from build123d import *

# Parameters (mm, degrees)
F0_W          = 6.5
F0_H          = 6.5
F1_DEPTH      = 10
F2_R          = 2.25
F3_DEPTH      = 2.5
F3_DEPTH_BACK = 12.5
F4_R          = 2.5
F5_DEPTH      = 25


with BuildPart() as f1:
    # F0 (on Front) → F1 (new body)
    with BuildSketch(Plane.XZ):
        with Locations((3.25, 3.25)):
            Rectangle(F0_W, F0_H)
    extrude(amount=F1_DEPTH)

    # F2 (on face) → F3 (join, two sides)
    with BuildSketch(Plane.XZ.offset(10)) as f3_sk:
        with Locations((3.25, 3.25)):
            Circle(F2_R)
    extrude(amount=F3_DEPTH)
    extrude(f3_sk.sketch, amount=-F3_DEPTH_BACK)

    # F4 (on face) → F5 (cut)
    with BuildSketch(Plane.YZ.offset(6.5)):
        with Locations((-5, 3.25)):
            Circle(F4_R)
    extrude(amount=-F5_DEPTH, mode=Mode.SUBTRACT)


solid = f1.part
Build history of the part. All positions in model axes, mm. A direction names the side the tool comes from. Round coordinates to 2 decimals unless told otherwise and drop trailing zeros. Write each loop counter-clockwise with the first axis right and the second up, starting at its lowest first coordinate (ties: lowest second). Pieces come first, ordered by that corner, then holes. Notation, with made-up numbers: (-9.75, 75.25) -> (11.25, 75.25) arc R23 ccw to (11.25, 86.25) -> close; hole circle Ø8 at (48, 87.25). An arc over 180 degrees is marked (long way). Use one line per item in the form item = value.
Q1. Band-saw the part on B-B, the plane y = -5. Write the cut outline in (x, z).
Conclusion:
outline = (0, 0) -> (6.5, 0) -> (6.5, 0.75) -> (0, 0.75) -> close; (0, 5.75) -> (6.5, 5.75) -> (6.5, 6.5) -> (0, 6.5) -> close
Q2. Tool access for faces 1 (the flat face through (2, -10, 1)), 2 (the flat face through (3, -5, 0)), 3 (the flat face through (2, 0, 1)): list every direction of +Z, -Z, +X, -X, +Y, -Y with a clear straight run to the whole face (end or side of a thin tool).
Conclusion:
face_1 = -Y
face_2 = -Z, +X, -X, +Y, -Y
face_3 = +Y
Q3. Band-saw the part on A-A, the plane x = 3.25. Write the cut outline in (y, z), then the cut area to 3 significant figures.
Conclusion:
outline = (-12.5, 1) -> (-10, 1) -> (-10, 0) -> (0, 0) -> (0, 1) -> (2.5, 1) -> (2.5, 5.5) -> (0, 5.5) -> (0, 6.5) -> (-10, 6.5) -> (-10, 5.5) -> (-12.5, 5.5) -> close; hole circle Ø5 at (-5, 3.25)
area = 67.9 mm²
Q4. Drop a flat-ended pin along its axis: P1, Ø1.5, axis at y = -5.5, z = 4, coming from the -X side. Give the stop position or say it passes through.
Conclusion:
P1 = through
Q5. Drill centre lines: L1, parallel to Z at x = 5.25, y = -5; L2, parallel to Y at x = 1, z = 4.5; L3, parallel to Z at x = 3.5, y = -7. Where is each one in solid material? Low to high.
Conclusion:
L1 = 0 to 0.75, 5.75 to 6.5
L2 = -10 to -7.17, -2.83 to 0
L3 = 0 to 1.75, 4.75 to 6.5
Q6. Band-saw the part on D-D, the plane z = 5. Write the cut outline in (x, y), then the cut area to 3 significant figures.
Conclusion:
outline = (0, -10) -> (1.84, -10) -> (1.84, -12.5) -> (4.66, -12.5) -> (4.66, -10) -> (6.5, -10) -> (6.5, -6.79) -> (0, -6.79) -> close; (0, -3.21) -> (6.5, -3.21) -> (6.5, 0) -> (4.66, 0) -> (4.66, 2.5) -> (1.84, 2.5) -> (1.84, 0) -> (0, 0) -> close
area = 55.9 mm²
Q7. Band-saw the part on C-C, the plane z = 3.25. Write the cut outline in (x, y).
Conclusion:
outline = (0, -10) -> (1, -10) -> (1, -12.5) -> (5.5, -12.5) -> (5.5, -10) -> (6.5, -10) -> (6.5, -7.5) -> (0, -7.5) -> close; (0, -2.5) -> (6.5, -2.5) -> (6.5, 0) -> (5.5, 0) -> (5.5, 2.5) -> (1, 2.5) -> (1, 0) -> (0, 0) -> close
